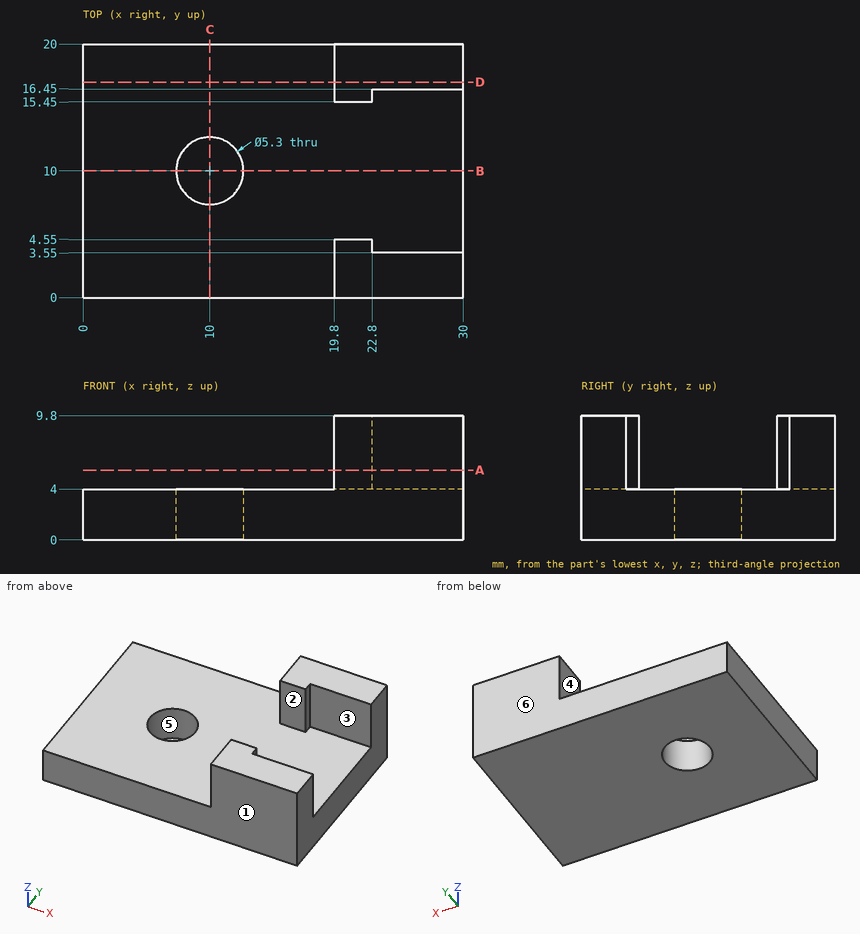
Part print with two shaded views. Sizes in mm from the minimum x, y, z corner. A direction names the side the tool comes from. Round coordinates to 2 decimals unless told otherwise and drop trailing zeros. Loops run counter-clockwise (first coordinate to the right, second up) from the corner with the lowest first, then second, coordinate; pieces in that order, holes last. Notation, with made-up numbers: M 71,44 L 108,44 A25 cw 108,57 Z; hole C 29.5,-4.75 d2. An arc over 180 degrees is marked long. Return JSON: item names as keys, results as strings. Group by question number.
(1) Saw through at A-A, the plane z = 5.5. List the corners of the cut face in (x, y), and give its area (3 significant figures).
(2) Drop flat-ended pins along their axis: P1, Ø2, axis at x = 9, z = 6.5, coming from the -Y side; P2, Ø4, axis at x = 15.5, y = 11, coming from the -Z side; P3, Ø1.5, axis at x = 11, y = 6, coming from the +Z side; P4, Ø0.8, axis at y = 16, z = 7.5, coming from the +X side. Give the stop position or say it passes through.
(3) Mould opens along Y. For the marked faces 4, 5 and 6 say: +Y half, -Y half, draft (parallel to the pull), parting line (faces both ways), or undercut.
(4) Saw through at B-B, the plane y = 10. List the corners of the cut face in (x, z), and give its area (3 significant figures).
(5) Wall check: probe 1 along Y at (x, z) = (10, 1.8); probe 2 along Z at (x, y) = (1.75, 11.25); probe 3 along Y at (x, z) = (28.5, 7). Give the ranges that are in metal, low to high. Write a range as [from, to].
(6) Saw through at C-C, the plane x = 10. List the corners of the cut face in (y, z), and give its area (3 significant figures).
(7) Tool access for the marked faces 1, 2 and 3: list every direction of +Z, -Z, +X, -X, +Y, -Y with a clear straight run to the whole face (end or side of a thin tool).
(8) Saw through at D-D, the plane y = 17. List the corners of the cut face in (x, z).
Answer list:
{
 "1": {"outline": "M 19.8,0 L 30,0 L 30,3.55 L 22.8,3.55 L 22.8,4.55 L 19.8,4.55 Z; M 19.8,15.45 L 22.8,15.45 L 22.8,16.45 L 30,16.45 L 30,20 L 19.8,20 Z", "area": "78.4 mm2"},
 "2": {"P1": "through", "P2": "z = 0", "P3": "z = 4", "P4": "x = 22.8"},
 "3": {"face 4": "draft", "face 5": "undercut", "face 6": "+Y half"},
 "4": {"outline": "M 0,0 L 7.35,0 L 7.35,4 L 0,4 Z; M 12.65,0 L 30,0 L 30,4 L 12.65,4 Z", "area": "98.8 mm2"},
 "5": {"probe 1": "[0, 7.35], [12.65, 20]", "probe 2": "[0, 4]", "probe 3": "[0, 3.55], [16.45, 20]"},
 "6": {"outline": "M 0,0 L 7.35,0 L 7.35,4 L 0,4 Z; M 12.65,0 L 20,0 L 20,4 L 12.65,4 Z", "area": "58.8 mm2"},
 "7": {"face 1": "+Z, -Z, +X, -X, -Y", "face 2": "+Z, +X, -X", "face 3": "+Z, +X"},
 "8": {"outline": "M 0,0 L 30,0 L 30,9.8 L 19.8,9.8 L 19.8,4 L 0,4 Z"}
}
